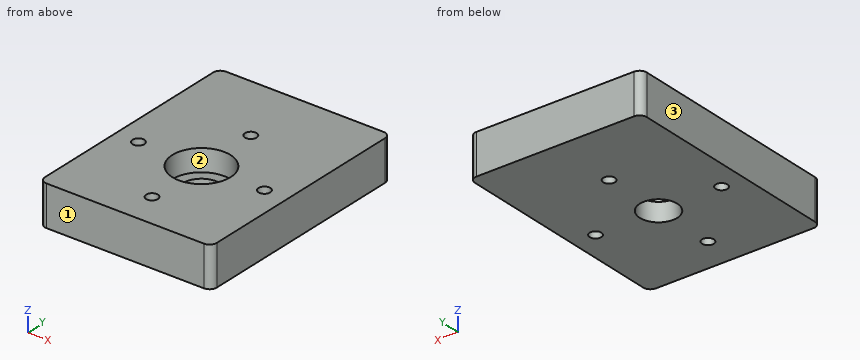
```python
from build123d import *

# Parameters (mm, degrees)
SKETCH1_W                                        = 30
SKETCH1_H                                        = 40
BOSS_EXTRUDE1_DEPTH                              = 7.0358
TAP_DRILL_FOR_M2_5X0_45_TAP1_D                   = 2.05
CBORE_FOR_1_4_SOCKET_HEAD_CAP_SCREW1_D           = 6.5278
CBORE_FOR_1_4_SOCKET_HEAD_CAP_SCREW1_CBORE_D     = 10.16
CBORE_FOR_1_4_SOCKET_HEAD_CAP_SCREW1_CBORE_DEPTH = 3.81
FILLET1_R                                        = 1.27


with BuildPart() as part:
    # Sketch1 → Boss-Extrude1 (new body)
    with BuildSketch(Plane.XY):
        with Locations((15, 20)):
            Rectangle(SKETCH1_W, SKETCH1_H)
    extrude(amount=BOSS_EXTRUDE1_DEPTH)

    # Tap Drill for M2.5x0.45 Tap1 (through all)
    with Locations(Plane.XY.offset(7.0358)):
        with Locations((15, 27.98), (26, 16.98), (15, 5.98), (4, 16.98)):
            Hole(TAP_DRILL_FOR_M2_5X0_45_TAP1_D / 2)

    # CBORE for 1/4 Socket Head Cap Screw1 (through all)
    with Locations(Plane.XY.offset(7.0358)):
        with Locations((15, 16.98)):
            CounterBoreHole(CBORE_FOR_1_4_SOCKET_HEAD_CAP_SCREW1_D / 2, CBORE_FOR_1_4_SOCKET_HEAD_CAP_SCREW1_CBORE_D / 2, CBORE_FOR_1_4_SOCKET_HEAD_CAP_SCREW1_CBORE_DEPTH)

    # Fillet1
    fillet1_edges = [part.edges().sort_by_distance(p)[0] for p in [
        (0, 40, 3.5179),
        (30, 40, 3.5179),
        (30, 0, 3.5179),
        (0, 0, 3.5179),
    ]]
    fillet(fillet1_edges, radius=FILLET1_R)


solid = part.part
```
Check sheet for the modelled part. Datum: model origin and axes. Units: mm. Face numbers are marked on the shaded views. Round coordinates to 2 decimals unless told otherwise and drop trailing zeros. Loops run counter-clockwise (first coordinate to the right, second up) from the corner with the lowest first, then second, coordinate; pieces in that order, holes last. Notation, with made-up numbers: (12.5, -8.5) - (38.5, -8.5) arc R24 ccw to (38.5, 20.5) - close; hole circle Ø10 at (-3.5, -19.5). An arc over 180 degrees is marked (long way). Write item = value, one per line. Start each with the question number.
Q1. Thickness scan on L1, parallel to Y at x = 15, z = 2.25 (3 decimals); L2, parallel to Y at x = 15, z = 4.75 (3 decimals); L3, parallel to Y at x = 4, z = 3 (3 decimals). Record the ranges inside material, lowest first.
Q2. Section check D-D (y = 27.98). Record the boundary of the cut face in (x, z) (3 decimals), plus the area to 3 significant figures.
Q3. Section check A-A (x = 26). Record the boundary of the cut face in (y, z) (3 decimals), plus the area to 3 significant figures.
Q4. Section check B-B (z = 1.75). Record the boundary of the cut face in (x, y) (3 decimals).
Q5. Section check C-C (y = 16.98). Record the boundary of the cut face in (x, z) (3 decimals).
Q6. Release check for a two-part mould opening along X. For the marked faces 1, 2 and 3 record: pulls with the +X half, pulls with the -X half, needs draft (parallel to the pull), parting line crosses it, or undercut.
Q7. Depth check by flat-ended pin: P1, Ø11, axis at x = 16, y = 16, coming from the +Z side; P2, Ø8, axis at x = 15, y = 16.98, coming from the +Z side. Enter the tip coordinate at first touch or a pass-through.
Derived:
q1.L1 = 0 to 4.955, 7.005 to 13.716, 20.244 to 26.955, 29.005 to 40
q1.L2 = 0 to 4.955, 7.005 to 11.9, 22.06 to 26.955, 29.005 to 40
q1.L3 = 0 to 15.955, 18.005 to 40
q2.outline = (0, 0) - (13.975, 0) - (13.975, 7.036) - (0, 7.036) - close; (16.025, 0) - (30, 0) - (30, 7.036) - (16.025, 7.036) - close
q2.area = 197 mm^2
q3.outline = (0, 0) - (15.955, 0) - (15.955, 7.036) - (0, 7.036) - close; (18.005, 0) - (40, 0) - (40, 7.036) - (18.005, 7.036) - close
q3.area = 267 mm^2
q4.outline = (0, 1.27) arc R1.27 ccw to (1.27, 0) - (28.73, 0) arc R1.27 ccw to (30, 1.27) - (30, 38.73) arc R1.27 ccw to (28.73, 40) - (1.27, 40) arc R1.27 ccw to (0, 38.73) - close; hole circle Ø2.05 at (4, 16.98); hole circle Ø6.528 at (15, 16.98); hole circle Ø2.05 at (15, 5.98); hole circle Ø2.05 at (15, 27.98); hole circle Ø2.05 at (26, 16.98)
q5.outline = (0, 0) - (2.975, 0) - (2.975, 7.036) - (0, 7.036) - close; (5.025, 0) - (11.736, 0) - (11.736, 3.226) - (9.92, 3.226) - (9.92, 7.036) - (5.025, 7.036) - close; (18.264, 0) - (24.975, 0) - (24.975, 7.036) - (20.08, 7.036) - (20.08, 3.226) - (18.264, 3.226) - close; (27.025, 0) - (30, 0) - (30, 7.036) - (27.025, 7.036) - close
q6.face_1 = needs draft
q6.face_2 = undercut
q6.face_3 = pulls with the -X half
q7.P1 = 7.04
q7.P2 = 3.23
